Check sheet for the modelled part. Datum: model origin and axes. Units: mm. Coordinates: 2 decimals unless noted, no trailing zeros. Loops run counter-clockwise (first coordinate to the right, second up) from the corner with the lowest first, then second, coordinate; pieces in that order, holes last. Notation, with made-up numbers: M 82.25,39.25 L 111.25,39.25 A19 cw 111.25,43.25 Z; hole C 79.5,45 d10. An arc over 180 degrees is marked long. Answer in a Markdown table with one row per item. Add a question column.
```python
from build123d import *

# Parameters (mm, degrees)
SKIZZE1_W                       = 250
SKIZZE1_H                       = 150
SKIZZE1_R                       = 12.5
AUFSATZ_LINEAR_AUSTRAGEN1_DEPTH = 10
VERRUNDUNG1_R                   = 10


with BuildPart() as part:
    # Skizze1 → Aufsatz-Linear austragen1 (new body)
    with BuildSketch(Plane.XY):
        Rectangle(SKIZZE1_W, SKIZZE1_H)
        Circle(SKIZZE1_R, mode=Mode.SUBTRACT)
    extrude(amount=AUFSATZ_LINEAR_AUSTRAGEN1_DEPTH)

    # Verrundung1
    verrundung1_edges = [part.edges().sort_by_distance(p)[0] for p in [
        (-125, 75, 5),
        (125, 75, 5),
        (125, -75, 5),
        (-125, -75, 5),
    ]]
    fillet(verrundung1_edges, radius=VERRUNDUNG1_R)


solid = part.part
```
Q1. Cross-section at C-C (z = 6.75). Record the cut outline in (x, y).
Q2. Mould release check, pull along Y, two halves, no side actions. Record for faces 1 (the face through (-122.15, 71.99, 5.07)), 2 (the face through (-2, 18, 0)), 3 (the face through (11.923, 3.755, 4.93)): released by +Y, released by -Y, zero draft, split by the parting line, or undercut.
Q3. Cross-section at B-B (x = 0). Record the cut outline in (y, z), plus the area to 3 significant figures.
Q4. Cross-section at A-A (y = 0). Record the cut outline in (x, z).
Q5. Thickness scan on L1, parallel to Y at x = 0, z = 3.5; L2, parallel to Y at x = 5.5, z = 9.5; L3, parallel to X at y = 5.5, z = 7. Record the ranges inside material, lowest first.
Answer key:
| question | item | result |
|---|---|---|
| 1 | outline | M -125,-65 A10 ccw -115,-75 L 115,-75 A10 ccw 125,-65 L 125,65 A10 ccw 115,75 L -115,75 A10 ccw -125,65 Z; hole C 0,0 d25 |
| 2 | face 1 | released by +Y |
| 2 | face 2 | zero draft |
| 2 | face 3 | undercut |
| 3 | outline | M -75,0 L -12.5,0 L -12.5,10 L -75,10 Z; M 12.5,0 L 75,0 L 75,10 L 12.5,10 Z |
| 3 | area | 1,250 mm^2 |
| 4 | outline | M -125,0 L -12.5,0 L -12.5,10 L -125,10 Z; M 12.5,0 L 125,0 L 125,10 L 12.5,10 Z |
| 5 | L1 | -75 to -12.5, 12.5 to 75 |
| 5 | L2 | -75 to -11.22, 11.22 to 75 |
| 5 | L3 | -125 to -11.22, 11.22 to 125 |
